Geometry: see drawing. Coordinates: mm, zero at the bounding-box minimum. Give positions to 0.01 mm unless a question says otherwise; leave off trailing zeros. Loops run counter-clockwise (first coordinate to the right, second up) from the corner with the lowest first, then second, coordinate; pieces in that order, holes last. Notation, with made-up numbers: (34.25, 24.25) -> (72.25, 24.25) arc R32 cw to (72.25, 57.25) -> close; hole circle Ø3 at (-14.5, 76.25). An arc over 180 degrees is marked (long way). One line per question, with ' | ' between items.
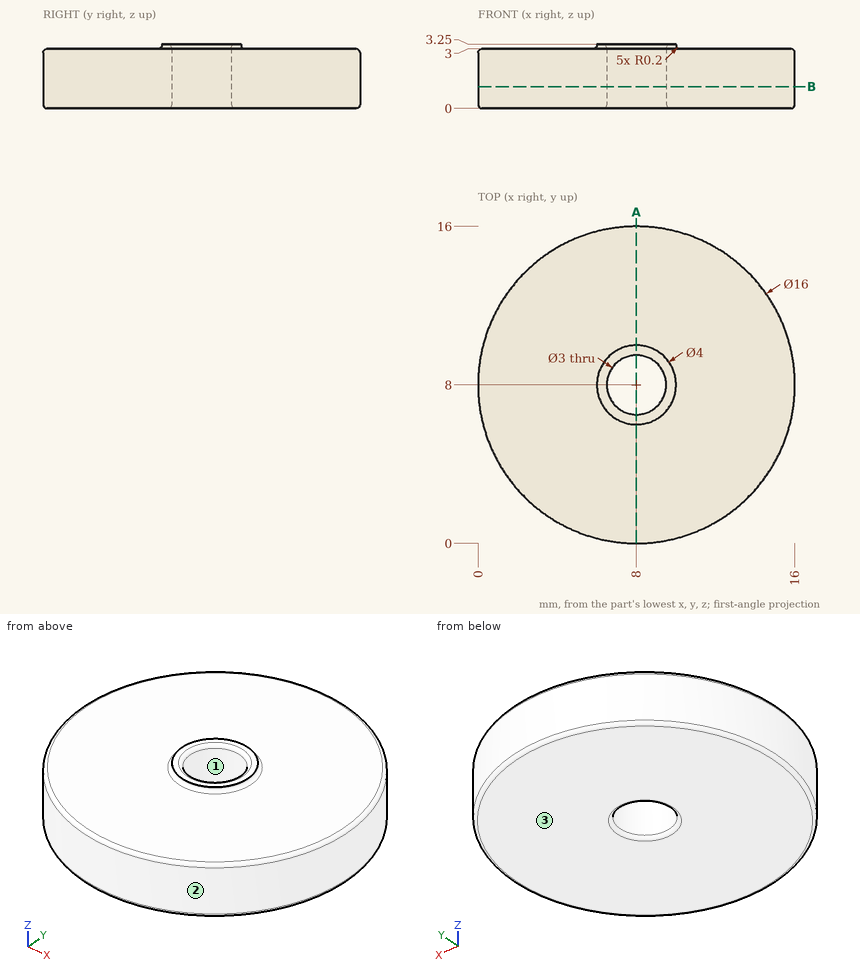
1. Section query A-A (x = 8). Output: boundary loops of the cut face in (y, z).
Determined:
outline: (0, 0.2) arc R0.2 ccw to (0.2, 0) -> (6.3, 0) arc R0.2 ccw to (6.5, 0.2) -> (6.5, 3.05) arc R0.2 ccw to (6.3, 3.25) -> (6, 3.25) -> (6, 3.2) arc R0.2 cw to (5.8, 3) -> (0.2, 3) arc R0.2 ccw to (0, 2.8) -> close; (9.5, 0.2) arc R0.2 ccw to (9.7, 0) -> (15.8, 0) arc R0.2 ccw to (16, 0.2) -> (16, 2.8) arc R0.2 ccw to (15.8, 3) -> (10.2, 3) arc R0.2 cw to (10, 3.2) -> (10, 3.25) -> (9.7, 3.25) arc R0.2 ccw to (9.5, 3.05) -> close
2. Ray query, line 1 along Y through (x, z) = (8, 1.7); line 2 along Z through (x, y) = (2.5, 3); line 3 along Y through (x, z) = (12.75, 0.5). Return the intervals inside material, ascending. Write a range as from..to.
Determined:
line 1: y = 0..6.5, 9.5..16 | line 2: z = 0..3 | line 3: y = 1.56..14.44
3. Pull-direction query (X, two-part tool) for the marked faces 1, 2 and 3; classes: pulls with the +X half, pulls with the -X half, needs draft (parallel to the pull), parting line crosses it, or undercut.
Determined:
face 1: undercut | face 2: parting line crosses it | face 3: needs draft
4. Section query B-B (z = 1.1). Output: boundary loops of the cut face in (x, y).
Determined:
outline: circle Ø16 at (8, 8); hole circle Ø3 at (8, 8)
5. Pin query (flat end, axial travel): P1, Ø1, axis at x = 5.5, z = 2.5, coming from the +Y side; P2, Ø1, axis at x = 2, z = 1, coming from the -Y side; P3, Ø1, axis at y = 12, z = 2, coming from the -X side; P4, Ø1.8, axis at x = 8, y = 8, coming from the -Z side. Return the tip coordinate at first contact, or that it passes through.
Determined:
P1: stops at y = 15.75 | P2: stops at y = 2.19 | P3: stops at x = 0.81 | P4: passes through
